```python
from build123d import *

# Parameters (mm, degrees)
SKETCH1_R           = 1.75
SKETCH1_R_2         = 2.7
BOSS_EXTRUDE1_DEPTH = 3
FILLET1_R           = 10


with BuildPart() as part:
    # Sketch1 → Boss-Extrude1 (new body)
    with BuildSketch(Plane.XY):
        Polygon((46.715728753, 141.715728753), (-75, 20), (-75, -20), (75, -20), (75, 20), (75, 113.431457505), align=None)
        with Locations((-65, -10)):
            Circle(SKETCH1_R, mode=Mode.SUBTRACT)
        with Locations((-65, 10)):
            Circle(SKETCH1_R, mode=Mode.SUBTRACT)
        with Locations((0, 10)):
            Circle(SKETCH1_R, mode=Mode.SUBTRACT)
        with Locations((-55.857864376, 25)):
            Circle(SKETCH1_R, mode=Mode.SUBTRACT)
        with Locations((-27.573593129, 25)):
            Circle(SKETCH1_R, mode=Mode.SUBTRACT)
        with Locations((0, -10)):
            Circle(SKETCH1_R, mode=Mode.SUBTRACT)
        with Locations((65, -10)):
            Circle(SKETCH1_R, mode=Mode.SUBTRACT)
        with Locations((65, 10)):
            Circle(SKETCH1_R, mode=Mode.SUBTRACT)
        with BuildLine():
            ThreePointArc((7.820236345, 19), (5.320236345, 21.5), (7.820236345, 24))
            Line((7.820236345, 24), (37.820236345, 24))
            ThreePointArc((37.820236345, 24), (40.320236345, 21.5), (37.820236345, 19))
            Line((37.820236345, 19), (7.820236345, 19))
        make_face(mode=Mode.SUBTRACT)
        with BuildLine():
            ThreePointArc((7.820236345, 35), (2.820236345, 40), (7.820236345, 45))
            Line((7.820236345, 45), (37.820236345, 45))
            ThreePointArc((37.820236345, 45), (42.820236345, 40), (37.820236345, 35))
            Line((37.820236345, 35), (7.820236345, 35))
        make_face(mode=Mode.SUBTRACT)
        with BuildLine():
            ThreePointArc((7.820236345, 56), (5.320236345, 58.5), (7.820236345, 61))
            Line((7.820236345, 61), (37.820236345, 61))
            ThreePointArc((37.820236345, 61), (40.320236345, 58.5), (37.820236345, 56))
            Line((37.820236345, 56), (7.820236345, 56))
        make_face(mode=Mode.SUBTRACT)
        with Locations((-3.535533906, 77.32233047)):
            Circle(SKETCH1_R, mode=Mode.SUBTRACT)
        with Locations((17.67766953, 70.251262658)):
            Circle(SKETCH1_R, mode=Mode.SUBTRACT)
        with Locations((65, 89.289321881)):
            Circle(SKETCH1_R_2, mode=Mode.SUBTRACT)
        with Locations((60.857864376, 113.431457505)):
            Circle(SKETCH1_R, mode=Mode.SUBTRACT)
        with Locations((46.715728753, 127.573593129)):
            Circle(SKETCH1_R, mode=Mode.SUBTRACT)
    extrude(amount=BOSS_EXTRUDE1_DEPTH)

    # Fillet1
    fillet1_edges = [part.edges().sort_by_distance(p)[0] for p in [
        (75, -20, 1.5),
        (-75, -20, 1.5),
        (-75, 20, 1.5),
        (46.715728753, 141.715728753, 1.5),
        (75, 113.431457505, 1.5),
    ]]
    fillet(fillet1_edges, radius=FILLET1_R)


solid = part.part
```
Work out the finished part from the listing and answer in its coordinate system (mm). A direction names the side the tool comes from. Round coordinates to 2 decimals unless told otherwise and drop trailing zeros. Loops run counter-clockwise (first coordinate to the right, second up) from the corner with the lowest first, then second, coordinate; pieces in that order, holes last. Notation, with made-up numbers: M -4.5,47 L 34.5,47 A26 ccw 34.5,70 Z; hole C -2,5 d9. An arc over 180 degrees is marked long. One line per question, with ' | ' between items.
Q1. The mould has two halves that part along Y. Classify faces 1 (the cylindrical face through (-63.331, -9.474, 1.479)), 2 (the flat face through (63.06, 125.37, 1.48)), 3 (the cylindrical face through (-72.15, -16.99, 1.52)), 4 (the flat face through (-1, 42, 0)): +Y half, -Y half, draft (parallel to the pull), parting line (faces both ways), or undercut.
Conclusion:
face 1: undercut | face 2: +Y half | face 3: -Y half | face 4: draft
Q2. Find section C-C, the plane y = 10. Give the vertices of the cut face in (x, z).
Conclusion:
outline: M -75,0 L -66.75,0 L -66.75,3 L -75,3 Z; M -63.25,0 L -1.75,0 L -1.75,3 L -63.25,3 Z; M 1.75,0 L 63.25,0 L 63.25,3 L 1.75,3 Z; M 66.75,0 L 75,0 L 75,3 L 66.75,3 Z
Q3. Find section A-A, the plane x = 0. Give the vertices of the cut face in (y, z), then the cut area to 3 significant figures.
Conclusion:
outline: M -20,0 L -11.75,0 L -11.75,3 L -20,3 Z; M -8.25,0 L 8.25,0 L 8.25,3 L -8.25,3 Z; M 11.75,0 L 95,0 L 95,3 L 11.75,3 Z | area: 324 mm2
Q4. Find section B-B, the plane y = 40. Give the vertices of the cut face in (x, z), then the cut area to 3 significant figures.
Conclusion:
outline: M -55,0 L 2.82,0 L 2.82,3 L -55,3 Z; M 42.82,0 L 75,0 L 75,3 L 42.82,3 Z | area: 270 mm2
Q5. A tool of negligible diameter and unlimited length cuts with its end or side. For faces 5 (the flat face through (-1, 42, 3)), 6 (the cylindrical face through (42.82, 40.11, 1.48)), from which of +Z, -Z, +X, -X, +Y, -Y can it reach the whole face along a straight path? Write none if from no direction.
Conclusion:
face 5: +Z, +X, -X, +Y, -Y | face 6: +Z, -Z
Q6. Each of these flat-tipped pins is pushed along its axis until it touches: pin 1 Ø4.5 at (x, y) = (-27.57, 25) entering from +Z; pin 2 Ø2 at (x, y) = (46.72, 127.57) entering from -Z; pin 3 Ø1 at (y, z) = (104, 0.5) entering from -X; pin 4 Ø0.9 at (x, z) = (23.5, 1) entering from +Y. Where does it stop, or does it pass through?
Conclusion:
pin 1: stops at z = 3 | pin 2: passes through | pin 3: stops at x = 8.5 | pin 4: stops at y = 118.95
Q7. Consider line 1 along Y through (x, z) = (47, 1.05); line 2 along Y through (x, z) = (1, 1.55); line 3 along Y through (x, z) = (65, 1.3). Determine where each line is inside the solid, lowest interval first. Write a range as from..to.
Conclusion:
line 1: y = -20..125.85, 129.3..137.57 | line 2: y = -20..-11.44, -8.56..8.56, 11.44..96 | line 3: y = -20..-11.75, -8.25..8.25, 11.75..86.59, 91.99..123.43
Q8. Find section D-D, the plane y = 103. Give the vertices of the cut face in (x, z).
Conclusion:
outline: M 8,0 L 75,0 L 75,3 L 8,3 Z
